Verification items for this drawing (mm, ordinates from the low corner). A direction names the side the tool comes from. Coordinates: 2 decimals unless noted, no trailing zeros. Loops run counter-clockwise (first coordinate to the right, second up) from the corner with the lowest first, then second, coordinate; pieces in that order, holes last. Notation, with made-up numbers: M -22.75,5 L 21.25,5 A12 cw 21.25,12 Z; hole C 15.5,40.5 d3. An arc over 180 degrees is marked long. Return JSON: item names as keys, results as strings.
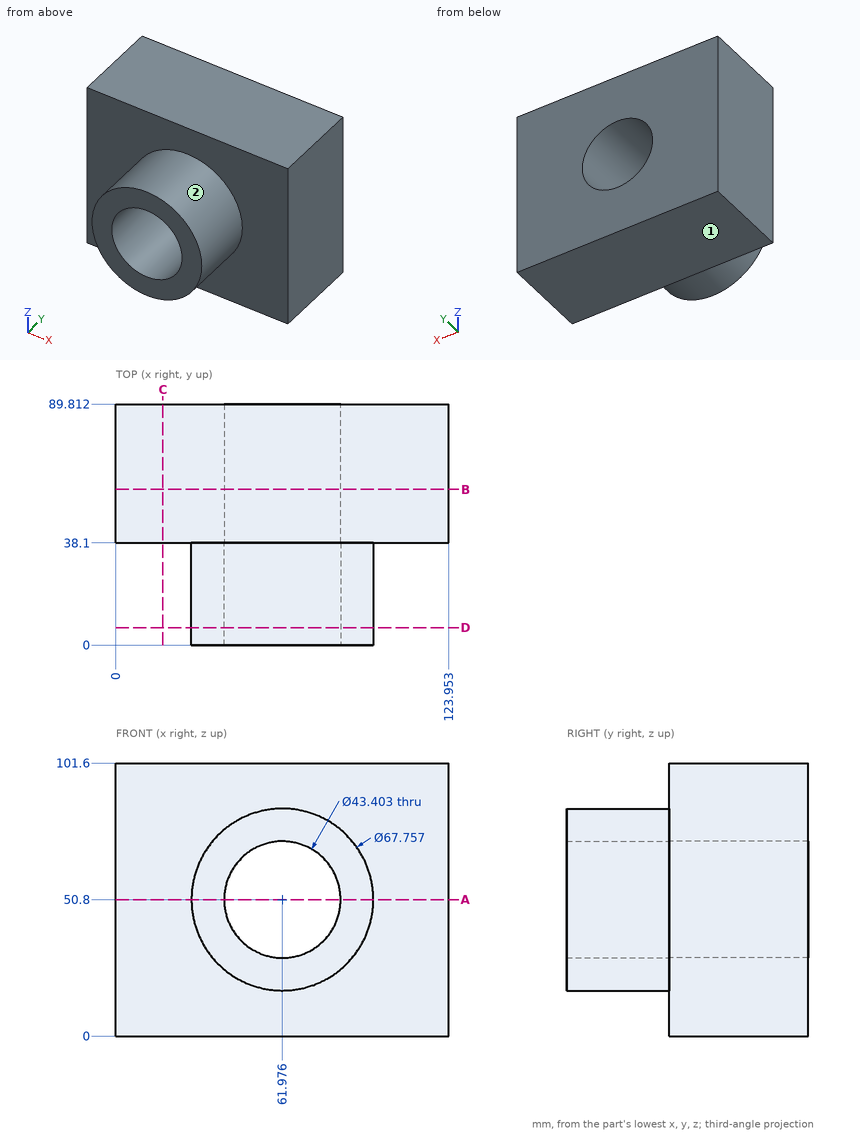
1) Section check B-B on y = 58. Record the cut outline in (x, z), then the cut area to 3 significant figures.
Answers:
{"outline": "M 0,0 L 123.95,0 L 123.95,101.6 L 0,101.6 Z; hole C 61.98,50.8 d43.4", "area": "11,100 mm²"}
2) Section check D-D on y = 6.5. Record the cut outline in (x, z) (1 decimal).
Answers:
{"outline": "C 62,50.8 d67.8; hole C 62,50.8 d43.4"}
3) Set-up check for the marked faces 1 and 2: record each of +Z, -Z, +X, -X, +Y, -Y from which the full face is reachable in a straight line by a thin tool's end or side.
Answers:
{"face 1": "-Z, +X, -X, +Y, -Y", "face 2": "-Y"}
4) Section check A-A on z = 50.8. Record the cut outline in (x, y) (1 decimal), then the cut area to 3 significant figures.
Answers:
{"outline": "M 0,38.1 L 28.1,38.1 L 28.1,0 L 40.3,0 L 40.3,89.8 L 0,89.8 Z; M 83.7,0 L 95.9,0 L 95.9,38.1 L 124,38.1 L 124,89.8 L 83.7,89.8 Z", "area": "5,090 mm²"}
5) Section check C-C on x = 17.5. Record the cut outline in (y, z), then the cut area to 3 significant figures.
Answers:
{"outline": "M 38.1,0 L 89.81,0 L 89.81,101.6 L 38.1,101.6 Z", "area": "5,250 mm²"}
6) Go/stop test with flat-tipped pins: pin 1 Ø10 at (y, z) = (26.5, 47) entering from +X (1 decimal); pin 2 Ø3 at (y, z) = (38.5, 37) entering from -X; pin 3 Ø6 at (x, y) = (51.5, 28) entering from +Z; pin 4 Ø12 at (x, z) = (73.5, 44.5) entering from -Y. Record where each tip stops, or that it passes through.
Answers:
{"pin 1": "x = 95.9", "pin 2": "x = 0", "pin 3": "z = 83.84", "pin 4": "through"}
7) Scan lines: line 1 along Y through (x, z) = (24, 79); line 2 along Z through (x, y) = (56, 5); line 3 along Z through (x, y) = (67.5, 30.5) (1 decimal). Record each from-to range of solid material in increasing order. Write a range as [from, to].
Answers:
{"line 1": "[38.1, 89.81]", "line 2": "[17.45, 29.94], [71.66, 84.15]", "line 3": "[17.4, 29.8], [71.8, 84.2]"}
